Source: CAD feature listing. Evaluate the final solid. Frame: model axes, mm. A direction names the side the tool comes from. Coordinates: 2 decimals unless noted, no trailing zeros. Order: outer loops, then holes, each group sorted by start corner. A loop starts at its lowest first (then second) coordinate and runs counter-clockwise, first axis right, second up.
```python
from build123d import *

# Parameters (mm, degrees)
F1_DEPTH = 30


with BuildPart() as f1:
    # F0 (on Front) → F1 (new body)
    with BuildSketch(Plane.XZ):
        with BuildLine():
            Line((-19.756784, 63.263963), (-119.756784, 63.263963))
            ThreePointArc((-119.756784, 63.263963), (-126.827851, 60.335031), (-129.756784, 53.263963))
            Line((-129.756784, 53.263963), (-129.756784, -86.736037))
            ThreePointArc((-129.756784, -86.736037), (-126.827851, -93.807104), (-119.756784, -96.736037))
            Line((-119.756784, -96.736037), (-19.756784, -96.736037))
            ThreePointArc((-19.756784, -96.736037), (-12.685716, -93.807104), (-9.756784, -86.736037))
            Line((-9.756784, -86.736037), (-9.756784, -76.736037))
            ThreePointArc((-9.756784, -76.736037), (-6.827851, -69.664969), (0.243216, -66.736037))
            Line((0.243216, -66.736037), (180.243216, -66.736037))
            ThreePointArc((180.243216, -66.736037), (187.314284, -63.807104), (190.243216, -56.736037))
            Line((190.243216, -56.736037), (190.243216, 23.263963))
            ThreePointArc((190.243216, 23.263963), (187.314284, 30.335031), (180.243216, 33.263963))
            Line((180.243216, 33.263963), (0.243216, 33.263963))
            ThreePointArc((0.243216, 33.263963), (-6.827851, 36.192896), (-9.756784, 43.263963))
            Line((-9.756784, 43.263963), (-9.756784, 53.263963))
            ThreePointArc((-9.756784, 53.263963), (-12.685716, 60.335031), (-19.756784, 63.263963))
        make_face()
        with BuildLine():
            ThreePointArc((-109.756784, -46.736037), (-106.827851, -39.664969), (-99.756784, -36.736037))
            Line((-99.756784, -36.736037), (-39.756784, -36.736037))
            ThreePointArc((-39.756784, -36.736037), (-32.685716, -39.664969), (-29.756784, -46.736037))
            Line((-29.756784, -46.736037), (-29.756784, -66.736037))
            ThreePointArc((-29.756784, -66.736037), (-32.685716, -73.807104), (-39.756784, -76.736037))
            Line((-39.756784, -76.736037), (-99.756784, -76.736037))
            ThreePointArc((-99.756784, -76.736037), (-106.827851, -73.807104), (-109.756784, -66.736037))
            Line((-109.756784, -66.736037), (-109.756784, -46.736037))
        make_face(mode=Mode.SUBTRACT)
        with BuildLine():
            ThreePointArc((-0.117784, -47.720788), (2.811149, -40.64972), (9.882216, -37.720788))
            Line((9.882216, -37.720788), (160.243216, -37.720788))
            ThreePointArc((160.243216, -37.720788), (167.314284, -40.64972), (170.243216, -47.720788))
            ThreePointArc((170.243216, -47.720788), (167.314284, -54.791856), (160.243216, -57.720788))
            Line((160.243216, -57.720788), (9.882216, -57.720788))
            ThreePointArc((9.882216, -57.720788), (2.811149, -54.791856), (-0.117784, -47.720788))
        make_face(mode=Mode.SUBTRACT)
        with BuildLine():
            ThreePointArc((-109.756784, 33.263963), (-106.827851, 40.335031), (-99.756784, 43.263963))
            Line((-99.756784, 43.263963), (-39.756784, 43.263963))
            ThreePointArc((-39.756784, 43.263963), (-32.685716, 40.335031), (-29.756784, 33.263963))
            Line((-29.756784, 33.263963), (-29.756784, 13.263963))
            ThreePointArc((-29.756784, 13.263963), (-32.685716, 6.192896), (-39.756784, 3.263963))
            Line((-39.756784, 3.263963), (-99.756784, 3.263963))
            ThreePointArc((-99.756784, 3.263963), (-106.827851, 6.192896), (-109.756784, 13.263963))
            Line((-109.756784, 13.263963), (-109.756784, 33.263963))
        make_face(mode=Mode.SUBTRACT)
        with BuildLine():
            ThreePointArc((-0.117784, -16.736037), (2.811149, -9.664969), (9.882216, -6.736037))
            Line((9.882216, -6.736037), (160.243216, -6.736037))
            ThreePointArc((160.243216, -6.736037), (167.314284, -9.664969), (170.243216, -16.736037))
            ThreePointArc((170.243216, -16.736037), (167.314284, -23.807104), (160.243216, -26.736037))
            Line((160.243216, -26.736037), (9.882216, -26.736037))
            ThreePointArc((9.882216, -26.736037), (2.811149, -23.807104), (-0.117784, -16.736037))
        make_face(mode=Mode.SUBTRACT)
        with BuildLine():
            ThreePointArc((-0.117468, 13.263963), (2.811464, 20.335031), (9.882532, 23.263963))
            Line((9.882532, 23.263963), (160.243216, 23.263963))
            ThreePointArc((160.243216, 23.263963), (167.314284, 20.335031), (170.243216, 13.263963))
            ThreePointArc((170.243216, 13.263963), (167.314284, 6.192896), (160.243216, 3.263963))
            Line((160.243216, 3.263963), (9.882532, 3.263963))
            ThreePointArc((9.882532, 3.263963), (2.811464, 6.192896), (-0.117468, 13.263963))
        make_face(mode=Mode.SUBTRACT)
    extrude(amount=F1_DEPTH)


solid = f1.part
```
Q1. Material intervals for line 1 along Z through (x, y) = (-69, -11.25); line 2 along Z through (x, y) = (30, -25); line 3 along X through (y, z) = (-22.25, -56.5), sorted ascending.
Solutions:
line 1: z = -96.74 to -76.74, -36.74 to 3.26, 43.26 to 63.26
line 2: z = -66.74 to -57.72, -37.72 to -26.74, -6.74 to 3.26, 23.26 to 33.26
line 3: x = -129.76 to -109.76, -29.76 to 5.09, 165.03 to 190.24
Q2. Section query D-D on y = -5.5. Give the number of separate pieces and of enclosed holes in the cut face, plus the area to 3 significant figures.
Solutions:
separate pieces: 1
enclosed holes: 5
area: 22,900 mm2
Q3. Section query A-A on x = 156. Output: boundary loops of the cut face in (y, z).
Solutions:
outline: (-30, -66.74) - (0, -66.74) - (0, -57.72) - (-30, -57.72) - close; (-30, -37.72) - (0, -37.72) - (0, -26.74) - (-30, -26.74) - close; (-30, -6.74) - (0, -6.74) - (0, 3.26) - (-30, 3.26) - close; (-30, 23.26) - (0, 23.26) - (0, 33.26) - (-30, 33.26) - close
Q4. Pin query (flat end, axial travel): P1, Ø1, axis at y = -13, z = 26.5, coming from the +X side; P2, Ø4, axis at x = 62.5, y = -17, coming from the +Z side; P3, Ø8, axis at y = -20.5, z = -82, coming from the +X side. Return the tip coordinate at first contact, or that it passes through.
Solutions:
P1: stops at x = 189.86
P2: stops at z = 33.26
P3: stops at x = -9.76
Q5. Set-up query: faces 4 (the flat face through (92, -15, 33.264)), 5 (the flat face through (86, -15, 3.264)), 6 (the cylindrical face through (-6.905, -14.79, -69.743)). Return all of +Z, -Z, +X, -X, +Y, -Y with unobstructed straight access to the full face (end or side cutting, diameter ignored); none if empty.
Solutions:
face 4: +Z, +X, +Y, -Y
face 5: +Y, -Y
face 6: -Z, +X, +Y, -Y
Q6. Pull-direction query (Z, two-part tool) for faces 1 (the cylindrical face through (-12.76, -14.79, -93.88)), 2 (the cylindrical face through (-126.75, -14.79, 60.41)), 3 (the flat face through (-29.757, -15, 23)); classes: pulls with the +Z half, pulls with the -Z half, needs draft (parallel to the pull), parting line crosses it, or undercut.
Solutions:
face 1: pulls with the -Z half
face 2: pulls with the +Z half
face 3: undercut
Q7. Section query B-B on z = 19. Output: boundary loops of the cut face in (x, y), plus the area to 3 significant figures.
Solutions:
outline: (-129.76, -30) - (-109.76, -30) - (-109.76, 0) - (-129.76, 0) - close; (-29.76, -30) - (1.69, -30) - (1.69, 0) - (-29.76, 0) - close; (168.43, -30) - (190.24, -30) - (190.24, 0) - (168.43, 0) - close
area: 2,200 mm2
Q8. Section query C-C on x = -50. Output: boundary loops of the cut face in (y, z).
Solutions:
outline: (-30, -96.74) - (0, -96.74) - (0, -76.74) - (-30, -76.74) - close; (-30, -36.74) - (0, -36.74) - (0, 3.26) - (-30, 3.26) - close; (-30, 43.26) - (0, 43.26) - (0, 63.26) - (-30, 63.26) - close
